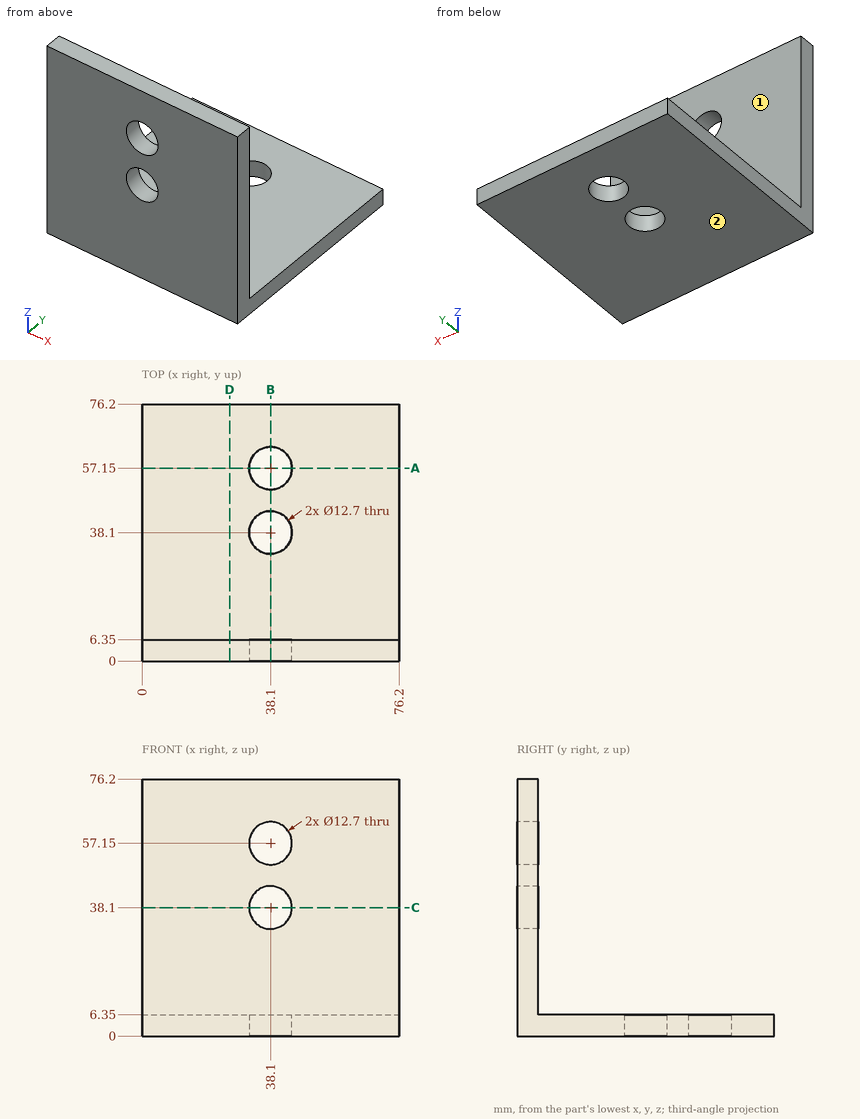
Print and shaded views of the part. All mm, measured from the part's lowest x, y and z. A direction names the side the tool comes from. Coordinates: 2 decimals unless noted, no trailing zeros. Write each loop counter-clockwise with the first axis right and the second up, starting at its lowest first coordinate (ties: lowest second). Pieces come first, ordered by that corner, then holes.
(1) Drill centre lines: probe 1 along Y at (x, z) = (38, 3); probe 2 along X at (y, z) = (3, 38). Where is each one in solid material? Low to high.
(2) 3-axis set-ups, long thin cutter, end or side, ignore diameter. For the marked faces 1 and 2: which of +Z, -Z, +X, -X, +Y, -Y reach the whole face in a straight line?
(3) Cut at B-B, the plane x = 38.1. List the corners of the cut face in (y, z).
(4) Flat gauge pins, fed straight in: pin 1 (6 mm diameter, centred on x = 61.5, y = 19.5, fed in from +Z); pin 2 (8 mm diameter, centred on x = 59.5, z = 66.5, fed in from +Y); pin 3 (10 mm diameter, centred on x = 61, z = 66.5, fed in from -Y). Where does each tip first touch, or does it go through?
(5) Cut at D-D, the plane x = 26. List the corners of the cut face in (y, z), and give its area (3 significant figures).
(6) Cut at A-A, the plane y = 57.15. List the corners of the cut face in (x, z), and give its area (3 significant figures).
Geometry says:
1. probe 1: y = 0 to 31.75, 44.45 to 50.8, 63.5 to 76.2
1. probe 2: x = 0 to 31.75, 44.45 to 76.2
2. face 1: +Z, +X, -X, +Y
2. face 2: -Z, +X, -X, +Y, -Y
3. outline: (0, 0) - (31.75, 0) - (31.75, 6.35) - (6.35, 6.35) - (6.35, 31.75) - (0, 31.75) - close; (0, 44.45) - (6.35, 44.45) - (6.35, 50.8) - (0, 50.8) - close; (0, 63.5) - (6.35, 63.5) - (6.35, 76.2) - (0, 76.2) - close; (44.45, 0) - (50.8, 0) - (50.8, 6.35) - (44.45, 6.35) - close; (63.5, 0) - (76.2, 0) - (76.2, 6.35) - (63.5, 6.35) - close
4. pin 1: stops at z = 6.35
4. pin 2: stops at y = 6.35
4. pin 3: stops at y = 0
5. outline: (0, 0) - (76.2, 0) - (76.2, 6.35) - (6.35, 6.35) - (6.35, 76.2) - (0, 76.2) - close
5. area: 927 mm2
6. outline: (0, 0) - (31.75, 0) - (31.75, 6.35) - (0, 6.35) - close; (44.45, 0) - (76.2, 0) - (76.2, 6.35) - (44.45, 6.35) - close
6. area: 403 mm2
